from build123d import *

# Parameters (mm, degrees)
SKETCH1_W               = 60
SKETCH1_H               = 60
SKETCH1_R               = 1.6
SKETCH1_W_2             = 12
SKETCH1_H_2             = 22
BOSS_EXTRUDE1_DEPTH     = 10
BOSS_EXTRUDE2_DEPTH     = 42
SKETCH3_R               = 11.5
CUT_EXTRUDE1_DEPTH      = 2
SKETCH4_R               = 8
CUT_EXTRUDE2_DEPTH      = 8
SKETCH5_R               = 1.6
CUT_EXTRUDE3_DEPTH      = 10
SKETCH6_R               = 3
CUT_EXTRUDE4_DEPTH      = 3
SKETCH7_R               = 3
CUT_EXTRUDE5_DEPTH      = 43
CUT_EXTRUDE6_DEPTH      = 31
CUT_EXTRUDE6_DEPTH_BACK = 31
FILLET1_R               = 2
FILLET2_R               = 2
CHAMFER1_SIZE           = 1


with BuildPart() as part:
    # Sketch1 → Boss-Extrude1 (new body)
    with BuildSketch(Plane(origin=(0, 0, 0), x_dir=(1, 0, 0), z_dir=(0, 1, 0))):
        Rectangle(SKETCH1_W, SKETCH1_H)
        with Locations((-22, 22)):
            Circle(SKETCH1_R, mode=Mode.SUBTRACT)
        with Locations((22, 22)):
            Circle(SKETCH1_R, mode=Mode.SUBTRACT)
        with Locations((-22, -22)):
            Circle(SKETCH1_R, mode=Mode.SUBTRACT)
        with Locations((22, -22)):
            Circle(SKETCH1_R, mode=Mode.SUBTRACT)
        Rectangle(SKETCH1_W_2, SKETCH1_H_2, mode=Mode.SUBTRACT)
    extrude(amount=BOSS_EXTRUDE1_DEPTH)

    # Sketch2 → Boss-Extrude2 (add)
    with BuildSketch(Plane(origin=(0, 10, 0), x_dir=(1, 0, 0), z_dir=(0, 1, 0))):
        Polygon((11, 30), (21, 30), (21, -30), (11, -30), (-14, -30), (-14, -25), (11, -25), (11, 25), (-14, 25), (-14, 30), align=None)
    extrude(amount=BOSS_EXTRUDE2_DEPTH)

    # Sketch3 → Cut-Extrude1 (cut)
    with BuildSketch(Plane(origin=(21, 0, 0), x_dir=(0, 0, -1), z_dir=(1, 0, 0))):
        with Locations((0, 31)):
            Circle(SKETCH3_R)
    extrude(amount=-CUT_EXTRUDE1_DEPTH, mode=Mode.SUBTRACT)

    # Sketch4 → Cut-Extrude2 (cut)
    with BuildSketch(Plane(origin=(19, 0, 0), x_dir=(0, 0, -1), z_dir=(1, 0, 0))):
        with Locations((0, 31)):
            Circle(SKETCH4_R)
    extrude(amount=-CUT_EXTRUDE2_DEPTH, mode=Mode.SUBTRACT)

    # Sketch5 → Cut-Extrude3 (cut)
    with BuildSketch(Plane(origin=(21, 0, 0), x_dir=(0, 0, -1), z_dir=(1, 0, 0))):
        with Locations((-15.5, 46.5)):
            Circle(SKETCH5_R)
        with Locations((15.5, 46.5)):
            Circle(SKETCH5_R)
        with Locations((15.5, 15.5)):
            Circle(SKETCH5_R)
        with Locations((-15.5, 15.5)):
            Circle(SKETCH5_R)
    extrude(amount=-CUT_EXTRUDE3_DEPTH, mode=Mode.SUBTRACT)

    # Sketch6 → Cut-Extrude4 (cut)
    with BuildSketch(Plane(origin=(0, 10, 0), x_dir=(1, 0, 0), z_dir=(0, 1, 0))):
        with Locations((-22, 22)):
            Circle(SKETCH6_R)
        with Locations((22, 22)):
            Circle(SKETCH6_R)
        with Locations((22, -22)):
            Circle(SKETCH6_R)
        with Locations((-22, -22)):
            Circle(SKETCH6_R)
    extrude(amount=-CUT_EXTRUDE4_DEPTH, mode=Mode.SUBTRACT)

    # Sketch7 → Cut-Extrude5 (cut, through all)
    with BuildSketch(Plane(origin=(0, 10, 0), x_dir=(1, 0, 0), z_dir=(0, 1, 0))):
        with Locations((22, 22)):
            Circle(SKETCH7_R)
        with Locations((22, -22)):
            Circle(SKETCH7_R)
    extrude(amount=CUT_EXTRUDE5_DEPTH, mode=Mode.SUBTRACT)

    # Sketch10 → Cut-Extrude6 (cut, two sides)
    with BuildSketch(Plane.XY) as cut_extrude6_sk:
        Polygon((11, 52), (-14, 10), (-19.679988527, 22.361973952), (-19.679988527, 54.584490378), (11, 54.584490378), align=None)
    extrude(amount=CUT_EXTRUDE6_DEPTH, mode=Mode.SUBTRACT)
    extrude(cut_extrude6_sk.sketch, amount=-CUT_EXTRUDE6_DEPTH_BACK, mode=Mode.SUBTRACT)

    # Fillet1
    fillet1_edges = [part.edges().sort_by_distance(p)[0] for p in [
        (21, 31, 30),
        (21, 31, -30),
        (-1.5, 10, -25),
        (11, 10, 0),
        (11, 31, -25),
        (-1.5, 10, 25),
        (11, 31, 25),
    ]]
    fillet(fillet1_edges, radius=FILLET1_R)

    # Fillet2
    fillet2_edges = [part.edges().sort_by_distance(p)[0] for p in [
        (30, 5, 30),
        (-30, 5, 30),
        (-30, 5, -30),
        (30, 5, -30),
    ]]
    fillet(fillet2_edges, radius=FILLET2_R)

    # Chamfer1
    chamfer1_edges = [part.edges().sort_by_distance(p)[0] for p in [
        (11, 31, 8),
    ]]
    chamfer(chamfer1_edges, length=CHAMFER1_SIZE)


solid = part.part
Part model, mm, in its own coordinate system. A direction names the side the tool comes from. Round coordinates to 2 decimals unless told otherwise and drop trailing zeros. Order: outer loops, then holes, each group sorted by start corner. A loop starts at its lowest first (then second) coordinate and runs counter-clockwise, first axis right, second up. Notation, with made-up numbers: (32.5, 14) -> (78.5, 14) arc R16 ccw to (78.5, 23) -> close; hole circle Ø3 at (8, 78). An arc over 180 degrees is marked (long way). Put each result on its own line as item: value.
Q1. Band-saw the part on D-D (y = 46.5). Give the cut face in (x, z).
From the geometry:
outline: (7.73, -30) -> (19, -30) arc R2 ccw to (21, -28) -> (21, -24.83) arc R3 cw to (21, -19.17) -> (21, -17.1) -> (11, -17.1) -> (11, -23) arc R2 cw to (9, -25) -> (7.73, -25) -> close; (7.73, 25) -> (9, 25) arc R2 cw to (11, 23) -> (11, 17.1) -> (21, 17.1) -> (21, 19.17) arc R3 cw to (21, 24.83) -> (21, 28) arc R2 ccw to (19, 30) -> (7.73, 30) -> close; (11, -13.9) -> (21, -13.9) -> (21, 13.9) -> (11, 13.9) -> close
Q2. Wall check: line 1 (Z direction, x = 22, y = 4); line 2 (X direction, y = 7.5, z = 9); line 3 (Y direction, x = 17, z = 15). Give the ranges that are in metal, low to high. Write a range as [from, to].
From the geometry:
line 1: z = [-30, -23.6], [-20.4, 20.4], [23.6, 30]
line 2: x = [-30, -6], [6, 30]
line 3: y = [0, 13.98], [17.02, 44.98], [48.02, 52]
Q3. Band-saw the part on B-B (y = 31). Give the cut face in (x, z), and give its area (4 significant figures).
From the geometry:
outline: (-1.5, -30) -> (19, -30) arc R2 ccw to (21, -28) -> (21, -24.83) arc R3 cw to (21, -19.17) -> (21, -11.5) -> (19, -11.5) -> (19, -8) -> (12, -8) -> (11, -9) -> (11, -23) arc R2 cw to (9, -25) -> (-1.5, -25) -> close; (-1.5, 25) -> (9, 25) arc R2 cw to (11, 23) -> (11, 9) -> (12, 8) -> (19, 8) -> (19, 11.5) -> (21, 11.5) -> (21, 19.17) arc R3 cw to (21, 24.83) -> (21, 28) arc R2 ccw to (19, 30) -> (-1.5, 30) -> close
area: 533.5 mm2
Q4. Pin check, flat tips, straight feed: pin 1 Ø5.5 at (x, z) = (-22, 22) entering from +Y; pin 2 Ø8 at (x, z) = (2.5, -12) entering from +Y; pin 3 Ø1.5 at (y, z) = (21, -8.5) entering from -X. Stop position of each tip, or through.
From the geometry:
pin 1: stops at y = 7
pin 2: stops at y = 10
pin 3: stops at x = 11
Q5. Band-saw the part on A-A (z = -22). Give the cut face in (x, y), and give its area (3 significant figures).
From the geometry:
outline: (-30, 0) -> (-23.6, 0) -> (-23.6, 7) -> (-25, 7) -> (-25, 10) -> (-30, 10) -> close; (-20.4, 0) -> (20.4, 0) -> (20.4, 7) -> (19, 7) -> (19, 52) -> (11, 52) -> (11, 12) arc R2 cw to (9, 10) -> (-19, 10) -> (-19, 7) -> (-20.4, 7) -> close; (23.6, 0) -> (30, 0) -> (30, 10) -> (25, 10) -> (25, 7) -> (23.6, 7) -> close
area: 856 mm2
Q6. Band-saw the part on C-C (x = -22.5). Give the cut face in (y, z), and give its area (3 significant figures).
From the geometry:
outline: (0, -30) -> (10, -30) -> (10, -24.96) -> (7, -24.96) -> (7, -23.52) -> (0, -23.52) -> close; (0, -20.48) -> (7, -20.48) -> (7, -19.04) -> (10, -19.04) -> (10, 19.04) -> (7, 19.04) -> (7, 20.48) -> (0, 20.48) -> close; (0, 23.52) -> (7, 23.52) -> (7, 24.96) -> (10, 24.96) -> (10, 30) -> (0, 30) -> close
area: 522 mm2
Q7. Tool access for faces 1 (the face through (0, 5, 11)), 2 (the face through (23.3, 7, 23.3)), 3 (the face through (20.4, 31.29, -29.43)), 4 (the face through (1, 26, -25)): list every direction of +Z, -Z, +X, -X, +Y, -Y with a clear straight run to the whole face (end or side of a thin tool).
From the geometry:
face 1: +Y, -Y
face 2: +Y
face 3: -Z, +X, +Y
face 4: -X, +Y
Q8. Pull direction Z, two halves, no side cores. Call faces 5 (the face through (-22.208, 3.451, 20.414)), 6 (the face through (26, 10, 0)), 7 (the face through (6, 20, 30)): pulls with the +Z half, pulls with the -Z half, needs draft (parallel to the pull), parting line crosses it, or undercut.
From the geometry:
face 5: undercut
face 6: needs draft
face 7: pulls with the +Z half
